Check sheet for the modelled part. Datum: model origin and axes. Units: mm. Face numbers are marked on the shaded views. A direction names the side the tool comes from. Coordinates: 2 decimals unless noted, no trailing zeros. Write each loop counter-clockwise with the first axis right and the second up, starting at its lowest first coordinate (ties: lowest second). Pieces come first, ordered by that corner, then holes. Notation, with made-up numbers: M 55,-1.5 L 110,-1.5 A15 ccw 110,24.5 Z; hole C 19.25,66 d8. An arc over 180 degrees is marked long. Answer as CSV lines item,"result".
from build123d import *

# Parameters (mm, degrees)
ESBO_O1_R                = 0.25
RESSALTO_EXTRUS_O1_DEPTH = 0.25
ESBO_O2_R                = 0.5
ESBO_O5_R                = 0.25
RESSALTO_EXTRUS_O2_DEPTH = 0.5
ESBO_O6_R                = 0.875
RESSALTO_EXTRUS_O3_DEPTH = 2
ESBO_O7_R                = 0.5
CORTE_EXTRUS_O1_DEPTH    = 2


with BuildPart() as part:
    # Esboço1 → Ressalto-extrusão1 (new body, symmetric)
    with BuildSketch(Plane(origin=(0, 0, 0), x_dir=(1, 0, 0), z_dir=(0, 1, 0))):
        with BuildLine():
            Line((-3.5, 0.5), (3.5, 0.5))
            ThreePointArc((3.5, 0.5), (4, 0), (3.5, -0.5))
            Line((3.5, -0.5), (-3.5, -0.5))
            ThreePointArc((-3.5, -0.5), (-4, 0), (-3.5, 0.5))
        make_face()
        with Locations((3.5, 0)):
            Circle(ESBO_O1_R, mode=Mode.SUBTRACT)
        with Locations((-3.5, 0)):
            Circle(ESBO_O1_R, mode=Mode.SUBTRACT)
        with BuildLine():
            Line((-1, 0.25), (1, 0.25))
            ThreePointArc((1, 0.25), (1.25, 0), (1, -0.25))
            Line((1, -0.25), (-1, -0.25))
            ThreePointArc((-1, -0.25), (-1.25, 0), (-1, 0.25))
        make_face(mode=Mode.SUBTRACT)
    extrude(amount=RESSALTO_EXTRUS_O1_DEPTH, both=True)

    # Varredura1: sweep along a path in Esboço3
    with BuildLine(Plane.XY) as varredura1_path:
        Line((-2.5, 0.25), (-2.5, 4.75))
        ThreePointArc((-2.5, 4.75), (0, 7.25), (2.5, 4.75))
        Line((2.5, 4.75), (2.5, 0.25))
    # Esboço2 → Varredura1 (sweep)
    with BuildSketch(Plane(origin=(0, 0.25, 0), x_dir=(1, 0, 0), z_dir=(0, 1, 0))):
        with Locations((-2.5, 0)):
            Circle(ESBO_O2_R)
    sweep(path=varredura1_path.line)

    # Esboço5 → Ressalto-extrusão2 (add, symmetric)
    with BuildSketch(Plane(origin=(-2.5, 0, 0), x_dir=(0, 0, -1), z_dir=(1, 0, 0))):
        with BuildLine():
            Line((0.5, -0.25), (-0.5, -0.25))
            Line((-0.5, -0.25), (-0.5, -1.25))
            ThreePointArc((-0.5, -1.25), (0, -1.75), (0.5, -1.25))
            Line((0.5, -1.25), (0.5, -0.25))
        make_face()
        with Locations((0, -1.25)):
            Circle(ESBO_O5_R, mode=Mode.SUBTRACT)
    ressalto_extrus_o2 = extrude(amount=RESSALTO_EXTRUS_O2_DEPTH, both=True)

    # Espelhar1: Ressalto-extrusão2 across plane
    add(ressalto_extrus_o2.mirror(Plane(origin=(0, 0, 0), x_dir=(0, 0, 1), z_dir=(1, 0, 0))))

    # Esboço6 → Ressalto-extrusão3 (add)
    with BuildSketch(Plane(origin=(0, 6, 0), x_dir=(1, 0, 0), z_dir=(0, 1, 0))):
        Circle(ESBO_O6_R)
    extrude(amount=RESSALTO_EXTRUS_O3_DEPTH)

    # Esboço7 → Corte-extrusão1 (cut)
    with BuildSketch(Plane(origin=(0, 8, 0), x_dir=(1, 0, 0), z_dir=(0, 1, 0))):
        Circle(ESBO_O7_R)
    extrude(amount=-CORTE_EXTRUS_O1_DEPTH, mode=Mode.SUBTRACT)


solid = part.part
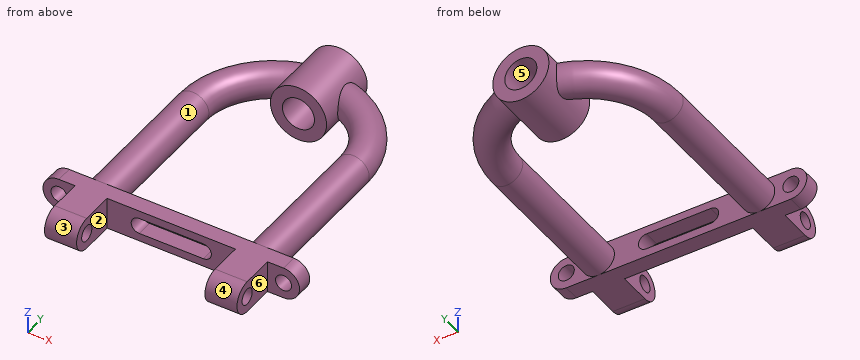
1) Mould release check, pull along X, two halves, no side actions. Record for the marked faces 4, 5 and 6: pulls with the +X half, pulls with the -X half, needs draft (parallel to the pull), parting line crosses it, or undercut.
Answer key:
face 4,"needs draft"
face 5,"undercut"
face 6,"pulls with the +X half"
2) Section check C-C, the plane z = 0. Give the number of separate pieces and of enclosed holes in the cut face, plus the area to 3 significant figures.
Answer key:
separate pieces,"6"
enclosed holes,"0"
area,"20.8 mm2"
3) Thickness scan on line 1 along Z through (x, y) = (-3.5, 0); line 2 along X through (y, z) = (6.25, -0.1); line 3 along X through (y, z) = (0, -0.05). Record the ranges inside material, lowest first.
Answer key:
line 1,"z = -0.5 to -0.25, 0.25 to 0.5"
line 2,"x = -2.59 to -1.34, -0.87 to -0.49, 0.49 to 0.87, 1.34 to 2.59"
line 3,"x = -4 to -3.74, -3.26 to -1.24, 1.24 to 3.26, 3.74 to 4"
4) Section check D-D, the plane z = -0.65. Record the boundary of the cut face in (x, y).
Answer key:
outline,"M -0.59,6 L 0.59,6 L 0.59,8 L -0.59,8 Z"
5) Section check B-B, the plane y = 2.5. Record the boundary of the cut face in (x, z).
Answer key:
outline,"C -2.5,0 d1; C 2.5,0 d1"
6) Depth check by flat-ended pin: P1, Ø1, axis at x = -2, y = 0.5, coming from the -Z side; P2, Ø0.8, axis at y = -1, z = 0, coming from the -X side; P3, Ø0.8, axis at y = -1, z = 0, coming from the +X side. Enter the tip coordinate at first touch or a pass-through.
Answer key:
P1,"stops at z = -0.5"
P2,"stops at x = -3"
P3,"stops at x = 3"
7) Tool access check on the marked faces 1, 2 and 3. Record the directions out of +Z, -Z, +X, -X, +Y, -Y that give a thin tool (end or side, any length) a straight path to the whole face; none if there is none.
Answer key:
face 1,"none"
face 2,"+Z, -Z, -Y"
face 3,"+X, -X, -Y"
8) Section check A-A, the plane x = -0.25. Record the boundary of the cut face in (y, z), plus the area to 3 significant figures.
Answer key:
outline,"M -0.25,-0.5 L 0.25,-0.5 L 0.25,-0.25 L -0.25,-0.25 Z; M -0.25,0.25 L 0.25,0.25 L 0.25,0.5 L -0.25,0.5 Z; M 6,-0.84 L 8,-0.84 L 8,-0.43 L 6,-0.43 Z; M 6,0.43 L 8,0.43 L 8,0.84 L 6,0.84 Z"
area,"1.87 mm2"
